Check sheet for the modelled part. Datum: model origin and axes. Units: mm. A direction names the side the tool comes from. Coordinates: 2 decimals unless noted, no trailing zeros. Write each loop counter-clockwise with the first axis right and the second up, starting at its lowest first coordinate (ties: lowest second). Pieces come first, ordered by that corner, then holes. Notation, with made-up numbers: (26.25, -31.5) -> (47.25, -31.5) arc R19 cw to (47.25, -19.5) -> close; hole circle Ø1 at (16.25, 32). An arc over 180 degrees is marked (long way). Put each result on its own line as item: value.
Autodesk Inventor part; units mm, degrees
ref_plane "YZ Plane" through (0, 0, 0) normal (1, 0, 0) x (0, 1, 0)
ref_plane "XZ Plane" through (0, 0, 0) normal (0, 1, 0) x (-1, 0, 0)
ref_plane "XY Plane" through (0, 0, 0) normal (0, 0, 1) x (1, 0, 0)
sketch "Sketch1" plane through (0, 0, 0) normal (0, 0, 1) x (1, 0, 0)
  line L0 (20.9262, 6.7683) -> (20.9262, 1.6883)
  line L1 (-14.6338, 1.6883) -> (-14.6338, 6.7683)
  line L2 (0.6062, 22.0083) -> (5.6862, 22.0083)
  line L3 (5.6862, -13.5517) -> (0.6062, -13.5517)
  line L4 (-3.2038, -9.7417) -> (-3.2038, -2.1217)
  line L5 (-3.2038, 10.5783) -> (-3.2038, 18.1983)
  line L6 (-10.8238, 10.5783) -> (-3.2038, 10.5783)
  line L7 (9.4962, 10.5783) -> (17.1162, 10.5783)
  line L8 (17.1162, -2.1217) -> (9.4962, -2.1217)
  line L9 (-3.2038, -2.1217) -> (-10.8238, -2.1217)
  line L10 (9.4962, 18.1983) -> (9.4962, 10.5783)
  line L11 (9.4962, -2.1217) -> (9.4962, -9.7417)
  line L12 (-3.2038, 18.1983) -> (0.6062, 22.0083)
  line L13 (5.6862, 22.0083) -> (9.4962, 18.1983)
  line L14 (17.1162, 10.5783) -> (20.9262, 6.7683)
  line L15 (20.9262, 1.6883) -> (17.1162, -2.1217)
  line L16 (9.4962, -9.7417) -> (5.6862, -13.5517)
  line L17 (-3.2038, -9.7417) -> (0.6062, -13.5517)
  line L18 (-14.6338, 1.6883) -> (-10.8238, -2.1217)
  line L19 (-14.6338, 6.7683) -> (-10.8238, 10.5783)
  line L20 (0.8602, 19.2143) -> (5.4322, 19.2143)
  line L21 (5.4322, 19.2143) -> (5.4322, 14.6423)
  line L22 (5.4322, 14.6423) -> (0.8602, 14.6423)
  line L23 (0.8602, 14.6423) -> (0.8602, 19.2143)
  line L24 (-11.8398, 6.5143) -> (-7.2678, 6.5143)
  line L25 (-7.2678, 6.5143) -> (-7.2678, 1.9423)
  line L26 (-7.2678, 1.9423) -> (-11.8398, 1.9423)
  line L27 (-11.8398, 1.9423) -> (-11.8398, 6.5143)
  line L28 (0.8602, -6.1857) -> (5.4322, -6.1857)
  line L29 (5.4322, -6.1857) -> (5.4322, -10.7577)
  line L30 (5.4322, -10.7577) -> (0.8602, -10.7577)
  line L31 (0.8602, -10.7577) -> (0.8602, -6.1857)
  line L32 (13.5602, 6.5143) -> (18.1322, 6.5143)
  line L33 (18.1322, 6.5143) -> (18.1322, 1.9423)
  line L34 (18.1322, 1.9423) -> (13.5602, 1.9423)
  line L35 (13.5602, 1.9423) -> (13.5602, 6.5143)
  line L36 (0.8602, 6.5143) -> (5.4322, 6.5143)
  line L37 (5.4322, 6.5143) -> (5.4322, 1.9423)
  line L38 (5.4322, 1.9423) -> (0.8602, 1.9423)
  line L39 (0.8602, 1.9423) -> (0.8602, 6.5143)
  point P0 (-14.6338, 10.5783)
  point P1 (20.9262, -2.1217)
  point P2 (20.9262, 10.5783)
  point P3 (-14.6338, -2.1217)
  point P4 (-3.2038, 22.0083)
  point P5 (9.4962, -13.5517)
  point P6 (9.4962, 22.0083)
  point P7 (-3.2038, -13.5517)
  dimension "d0" = 35.56
  dimension "d1" = 35.56
  dimension "d2" = 12.7
  dimension "d3" = 12.7
  dimension "d4" = 12.7
  dimension "d5" = 12.7
  dimension "d6" = 11.43
  dimension "d7" = 11.43
  dimension "d8" = 11.43
  dimension "d9" = 11.43
  dimension "d10" = 3.81
  dimension "d11" = 3.81
  dimension "d12" = 3.81
  dimension "d13" = 3.81
  dimension "d14" = 3.81
  dimension "d15" = 3.81
  dimension "d16" = 3.81
  dimension "d17" = 3.81
  dimension "d18" = 3.81
  dimension "d19" = 3.81
  dimension "d20" = 3.81
  dimension "d21" = 3.81
  dimension "d22" = 3.81
  dimension "d23" = 3.81
  dimension "d24" = 3.81
  dimension "d25" = 3.81
  dimension "d26" = 4.572
  dimension "d27" = 4.572
  dimension "d28" = 4.572
  dimension "d29" = 4.572
  dimension "d30" = 4.572
  dimension "d31" = 4.572
  dimension "d32" = 4.572
  dimension "d33" = 4.572
  dimension "d34" = 4.572
  dimension "d35" = 4.572
  dimension "d36" = 2.794
  dimension "d37" = 2.794
  dimension "d38" = 2.794
  dimension "d39" = 2.794
  dimension "d40" = 4.064
  dimension "d41" = 4.064
  dimension "d42" = 11.43
extrude "Extrusion1" add sketch "Sketch1" along normal blind 0.8382
sketch "Sketch2" plane through (0, 0, 0.8382) normal (0, 0, 1) x (1, 0, 0)
  line L0 (5.4322, 19.2143) -> (5.4322, 14.6423)
  line L1 (5.4322, 14.6423) -> (0.8602, 14.6423)
  line L2 (0.8602, 14.6423) -> (0.8602, 19.2143)
  line L3 (0.8602, 19.2143) -> (5.4322, 19.2143)
  circle A0 centre (3.1462, 16.9283) radius 2.286
  point P0 (0, 0)
surface extrude "ExtrusionSrf1" sketch "Sketch2" against normal up to surface (0.8382 mm away) shown no curves A0
pattern_linear "Rectangular Pattern1" count 3 spacing 12.7 along (0, -1, 0) of "ExtrusionSrf1"
sketch "Sketch3" plane through (0, 0, 0.8382) normal (0, 0, 1) x (1, 0, 0)
  line L0 (-7.2678, 6.5143) -> (-7.2678, 1.9423)
  line L1 (-7.2678, 1.9423) -> (-11.8398, 1.9423)
  line L2 (-11.8398, 1.9423) -> (-11.8398, 6.5143)
  line L3 (-11.8398, 6.5143) -> (-7.2678, 6.5143)
  circle A0 centre (-9.5538, 4.2283) radius 2.286
  point P0 (0, 0)
surface extrude "ExtrusionSrf4" sketch "Sketch3" against normal up to surface (0.8382 mm away) shown no curves A0
pattern_linear "Rectangular Pattern2" count 2 spacing 25.4 along (1, 0, 0) of "ExtrusionSrf4"
properties part number "276-1110" material "Steel"
Q1. Cross-section at B-B (x = 15.5). Record the cut outline in (y, z).
Recorded:
outline: (-2.12, 0) -> (1.94, 0) -> (1.94, 0.84) -> (-2.12, 0.84) -> close; (6.51, 0) -> (10.58, 0) -> (10.58, 0.84) -> (6.51, 0.84) -> close
Q2. Cross-section at C-C (z = 0.15). State how many separate pieces and enclosed holes the cut face has, plus the area to 3 significant figures.
Recorded:
separate pieces: 1
enclosed holes: 5
area: 579 mm2
Q3. Mould release check, pull along Y, two halves, no side actions. Record for faces 1 (the flat face through (-14.634, 4.2, 0.4)), 2 (the flat face through (19.05, -0.19, 0.41)), 3 (the flat face through (-9.6, 6.514, 0.4)): released by +Y, released by -Y, zero draft, split by the parting line, or undercut.
Recorded:
face 1: zero draft
face 2: released by -Y
face 3: undercut
Q4. Material ranges on line 1 along X through (y, z) = (-8, 0.7); line 2 along Y through (x, z) = (-10.5, 0.5); line 3 along X through (y, z) = (6, 0.25), recorded low to high.
Recorded:
line 1: x = -3.2 to 0.86, 5.43 to 9.5
line 2: y = -2.12 to 1.94, 6.51 to 10.58
line 3: x = -14.63 to -11.84, -7.27 to 0.86, 5.43 to 13.56, 18.13 to 20.93
Q5. Cross-section at D-D (y = 14). Record the cut outline in (x, z), plus the area to 3 significant figures.
Recorded:
outline: (-3.2, 0) -> (9.5, 0) -> (9.5, 0.84) -> (-3.2, 0.84) -> close
area: 10.6 mm2
Q6. Cross-section at A-A (y = -8.5). Record the cut outline in (x, z), plus the area to 3 significant figures.
Recorded:
outline: (-3.2, 0) -> (0.86, 0) -> (0.86, 0.84) -> (-3.2, 0.84) -> close; (5.43, 0) -> (9.5, 0) -> (9.5, 0.84) -> (5.43, 0.84) -> close
area: 6.81 mm2
Q7. Tool access check on faces 4 (the flat face through (9.496, 14.4, 0.4)), 5 (the flat face through (3, 8, 0.838)), 6 (the flat face through (15.9, 1.942, 0.4)). Record the directions out of +Z, -Z, +X, -X, +Y, -Y that give a thin tool (end or side, any length) a straight path to the whole face; none if there is none.
Recorded:
face 4: +Z, -Z, +X, +Y
face 5: +Z, +X, -X, +Y, -Y
face 6: +Z, -Z
